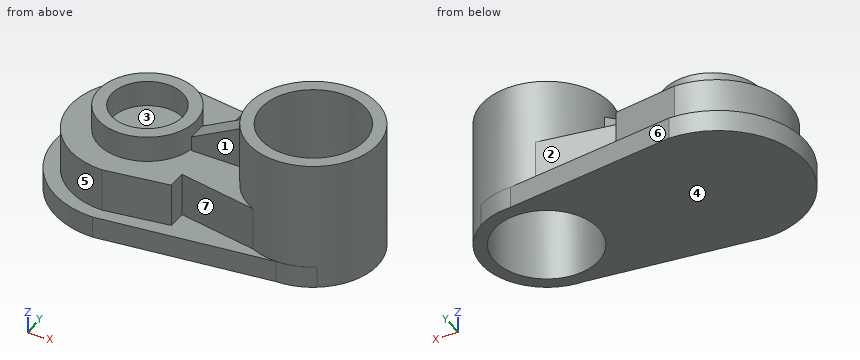
from build123d import *

# Parameters (mm, degrees)
F5_DEPTH  = 5
F1_R      = 14.9315093154
F6_DEPTH  = 30
F7_DEPTH  = 15
F3_R      = 11.3082404675
F3_R_2    = 8.2715191878
F8_DEPTH  = 21
F4_W      = 12.3962298967
F4_H      = 4.3726625154
F9_DEPTH  = 25
F11_DEPTH = 25
F12_R     = 12.0111757901
F13_DEPTH = 30


with BuildPart() as f5:
    # F0 (on Top) → F5 (new body)
    with BuildSketch(Plane.XY):
        with BuildLine():
            Line((8.6091840267, 15), (-31.3908159733, 20))
            ThreePointArc((-31.3908159733, 20), (-51.3908159733, 0), (-31.3908159733, -20))
            Line((-31.3908159733, -20), (8.6091840267, -15))
            ThreePointArc((8.6091840267, -15), (23.6091840267, 0), (8.6091840267, 15))
        make_face()
    extrude(amount=F5_DEPTH)

    # F1 (on face) → F6 (join)
    with BuildSketch(Plane.XY):
        with Locations((8.7348353118, 0)):
            Circle(F1_R)
    extrude(amount=F6_DEPTH)

    # F2 (on face) → F7 (join)
    with BuildSketch(Plane.XY):
        with BuildLine():
            Line((-16.0241960241, 14.8374513995), (-30.8759714769, 16.9409641518))
            ThreePointArc((-30.8759714769, 16.9409641518), (-47.8169356288, 0), (-30.8759714769, -16.9409641518))
            Line((-30.8759714769, -16.9409641518), (-16.060320359, -14.596506442))
            Line((-16.060320359, -14.596506442), (-16.060320359, -10.236135684))
            Line((-16.060320359, -10.236135684), (8.4618721157, -14.596506442))
            Line((8.4618721157, -14.596506442), (9.0077994391, 14.8374513995))
            Line((9.0077994391, 14.8374513995), (-16.0241960241, 10.782062076))
            Line((-16.0241960241, 10.782062076), (-16.0241960241, 14.8374513995))
        make_face()
    extrude(amount=F7_DEPTH)

    # F3 (on face) → F8 (join)
    with BuildSketch(Plane.XY):
        with Locations((-30.0259981304, 0)):
            Circle(F3_R)
        with Locations((-30.0259981304, 0)):
            Circle(F3_R_2, mode=Mode.SUBTRACT)
    extrude(amount=F8_DEPTH)

    # F4 (on face) → F9 (join)
    with BuildSketch(Plane.XY):
        with Locations((-12.3634112533, 0.1391041442)):
            Rectangle(F4_W, F4_H)
    extrude(amount=F9_DEPTH)

    # F10 (on face) → F11 (cut)
    with BuildSketch(Plane.XZ.offset(2.0472271135)):
        Polygon((-18.5615262017, 18.3737631887), (-6.165296305, 25), (-18.5615262017, 25), align=None)
    extrude(amount=-F11_DEPTH, mode=Mode.SUBTRACT)

    # F12 (on face) → F13 (cut)
    with BuildSketch(Plane.XY.offset(30)):
        with Locations((8.7348353118, 0)):
            Circle(F12_R)
    extrude(amount=-F13_DEPTH, mode=Mode.SUBTRACT)


solid = f5.part
The model under review builds one solid part; all positions refer to its coordinate system, in mm. Face numbers are marked on the shaded views. A direction names the side the tool comes from. Coordinates: 2 decimals unless noted, no trailing zeros. Loops run counter-clockwise (first coordinate to the right, second up) from the corner with the lowest first, then second, coordinate; pieces in that order, holes last. Notation, with made-up numbers: (45.25, 59.25) -> (79.25, 59.25) arc R26 ccw to (79.25, 88.25) -> close; hole circle Ø2 at (-36.5, 58). An arc over 180 degrees is marked (long way). Use a Markdown table: item, result. Add a question column.
1. Clearance check with flat-ended pins moving along their axes: pin 1 Ø1.5 at (x, y) = (-14.5, -7) entering from +Z; pin 2 Ø1.1 at (y, z) = (2, 21) entering from +X; pin 3 Ø12 at (x, y) = (-30, -3) entering from +Z; pin 4 Ø19 at (x, y) = (8.73, 0) entering from +Z. State where each tip first meets the part, or that it passes through.
2. Add section B-B on z = 8.75. Write out the cut boundary in (x, y).
3. To check wall thickness, follow line 1 (X direction, y = -3, z = 18.25); line 2 (X direction, y = -4, z = 16.5); line 3 (Y direction, x = 17.5, z = 26.25). State the ranges of each line that lie inside material, in increasing order.
4. Draft analysis for pull direction X (two halves, no side actions). For the marked faces 4, 5, 6 and 7, state which applies: pulls with the +X half, pulls with the -X half, needs draft (parallel to the pull), parting line crosses it, or undercut.
5. Machinability: for the marked faces 1, 2 and 3, which of the approach directions +Z, -Z, +X, -X, +Y, -Y give a long, thin tool a straight path to every point of the face, cutting with its end or side? Answer none if there is none.
6. Add section D-D on y = -5.5. Write out the cut boundary in (x, z).
7. Add section C-C on x = -14. Write out the cut boundary in (y, z).
Returned:
| question | item | result |
|---|---|---|
| 1 | pin 1 | stops at z = 15 |
| 1 | pin 2 | stops at x = 23.6 |
| 1 | pin 3 | stops at z = 21 |
| 1 | pin 4 | passes through |
| 2 | outline | (-30.88, -16.94) -> (-16.06, -14.6) -> (-16.06, -10.24) -> (2.39, -13.52) arc R14.93 ccw (long way) to (3.32, 13.92) -> (-16.02, 10.78) -> (-16.02, 14.84) -> (-30.88, 16.94) arc R16.94 ccw to start; hole circle Ø24.02 at (8.73, 0) |
| 3 | line 1 | x = -40.93 to -37.73, -22.32 to -19.12, -5.89 to -2.9, 20.37 to 23.36 |
| 3 | line 2 | x = -40.6 to -37.27, -22.79 to -19.45, -5.65 to -2.59, 20.06 to 23.12 |
| 3 | line 3 | y = -12.09 to -8.21, 8.21 to 12.09 |
| 4 | face 4 | needs draft |
| 4 | face 5 | pulls with the -X half |
| 4 | face 6 | pulls with the +X half |
| 4 | face 7 | undercut |
| 5 | face 1 | +Z, -Y |
| 5 | face 2 | +Z, +Y |
| 5 | face 3 | +Z |
| 6 | outline | (-50.62, 0) -> (-1.94, 0) -> (-1.94, 30) -> (-5.15, 30) -> (-5.15, 15) -> (-20.15, 15) -> (-20.15, 21) -> (-23.85, 21) -> (-23.85, 15) -> (-36.2, 15) -> (-36.2, 21) -> (-39.91, 21) -> (-39.91, 15) -> (-46.9, 15) -> (-46.9, 5) -> (-50.62, 5) -> close; (19.41, 0) -> (22.62, 0) -> (22.62, 30) -> (19.41, 30) -> close |
| 7 | outline | (-17.83, 0) -> (17.83, 0) -> (17.83, 5) -> (11.11, 5) -> (11.11, 15) -> (2.33, 15) -> (2.33, 20.81) -> (-2.05, 20.81) -> (-2.05, 15) -> (-10.6, 15) -> (-10.6, 5) -> (-17.83, 5) -> close |
